Could you check a few things on this model? Use its own coordinates, in mm. A direction names the side the tool comes from. Round coordinates to 2 decimals unless told otherwise and drop trailing zeros. Loops run counter-clockwise (first coordinate to the right, second up) from the corner with the lowest first, then second, coordinate; pieces in that order, holes last. Notation, with made-up numbers: (46.25, 52.25) -> (67.25, 52.25) arc R12 cw to (67.25, 65.25) -> close; hole circle Ø7 at (9, -35.75). An arc over 180 degrees is marked (long way). One line per item, written item: value.
Autodesk Fusion 360 part; units mm, degrees
sketch "Skizze1" plane through (0, 0, 0) normal (0, 0, 1) x (1, 0, 0)
  line L0 (-90, -60) -> (90, -60)
  line L1 (90, -60) -> (90, 60)
  line L2 (90, 60) -> (-90, 60)
  line L3 (-90, 60) -> (-90, -60)
  line L4 (0, -120.4862) -> (0, 94.8054) construction
  line L5 (-128.125, 0) -> (128.8109, 0) construction
  line L6 (-75, 45) -> (75, 45)
  line L7 (75, 45) -> (75, -45)
  line L8 (75, -45) -> (-75, -45)
  line L9 (-75, -45) -> (-75, 45)
  point P0 (0, 60)
  point P1 (-90, 0)
  point P2 (-75, 45)
  point P3 (75, 45)
  point P4 (75, -45)
  point P5 (-75, -45)
  dimension "d1" = 120
  dimension "d2" = 180
  dimension "d3" = 15
  dimension "d4" = 15
  dimension "d5" = 15
  dimension "d6" = 15
extrude "Extrusion1" add sketch "Skizze1" along normal blind 50 contours L0 L1 L2 L3 | L6 L7 L8 L9
sketch "Skizze2" plane through (0, 0, 50) normal (0, 0, 1) x (-1, 0, 0)
  line L0 (90, -60) -> (90, 60)
  line L1 (90, 60) -> (-90, 60)
  line L2 (-90, 60) -> (-90, -60)
  line L3 (-90, -60) -> (90, -60)
  point P0 (-75, 45)
  point P1 (-75, -45)
  point P2 (75, -45)
  point P3 (75, 45)
hole "Bohrung1" at (-75, 45, 50) at (-75, -45, 50) at (75, -45, 50) at (75, 45, 50) direction (0, 0, -1) diameter 6.6 depth 50 tip angle 180 counterbore diameter 14.55 counterbore depth 40
(1) For pin 1 Ø8.5 at (x, y) = (75, 45) entering from -Z; pin 2 Ø7.5 at (x, y) = (74.5, 44) entering from +Z, each with a flat end and sliding along its axis, tell me the tip position at first contact or that it passes through.
Results below:
pin 1: stops at z = 0
pin 2: stops at z = 10
(2) Imagine slicing it at C-C on x = -75. Write out the boundary of the cut face in (y, z) (3 decimals), then the cut area to 3 significant figures.
Results below:
outline: (-60, 0) -> (-48.3, 0) -> (-48.3, 10) -> (-52.275, 10) -> (-52.275, 50) -> (-60, 50) -> close; (-41.7, 0) -> (41.7, 0) -> (41.7, 10) -> (37.725, 10) -> (37.725, 50) -> (-37.725, 50) -> (-37.725, 10) -> (-41.7, 10) -> close; (48.3, 0) -> (60, 0) -> (60, 50) -> (52.275, 50) -> (52.275, 10) -> (48.3, 10) -> close
area: 4,700 mm²
(3) We'd pull the mould along Y, two halves only. Please class faces 3 (the face through (-1, -60, 25)), 4 (the face through (1, 60, 25)), 5 (the face through (-73, 42, 10)), 6 (the face through (-1, 1, 50)): +Y half, -Y half, draft (parallel to the pull), parting line (faces both ways), or undercut.
Results below:
face 3: -Y half
face 4: +Y half
face 5: undercut
face 6: draft
(4) Imagine slicing it at B-B on z = 37.5. Write out the boundary of the cut face in (x, y) (3 decimals), then the cut area to 3 significant figures.
Results below:
outline: (-90, -60) -> (90, -60) -> (90, 60) -> (-90, 60) -> close; hole circle Ø14.55 at (-75, -45); hole circle Ø14.55 at (-75, 45); hole circle Ø14.55 at (75, -45); hole circle Ø14.55 at (75, 45)
area: 20,900 mm²
(5) Imagine slicing it at A-A on y = -45. Write out the boundary of the cut face in (x, z) (3 decimals), then the cut area to 3 significant figures.
Results below:
outline: (-90, 0) -> (-78.3, 0) -> (-78.3, 10) -> (-82.275, 10) -> (-82.275, 50) -> (-90, 50) -> close; (-71.7, 0) -> (71.7, 0) -> (71.7, 10) -> (67.725, 10) -> (67.725, 50) -> (-67.725, 50) -> (-67.725, 10) -> (-71.7, 10) -> close; (78.3, 0) -> (90, 0) -> (90, 50) -> (82.275, 50) -> (82.275, 10) -> (78.3, 10) -> close
area: 7,700 mm²
(6) On a 3-axis mill with a long thin cutter (end or side, diameter ignored), from which of +Z, -Z, +X, -X, +Y, -Y can I reach the whole of each face in a straight line? I mean faces 1 (the face through (77, -48, 10)), 2 (the face through (-77.23, 47.43, 4.93)). Say none if no direction works.
Results below:
face 1: +Z
face 2: +Z, -Z
(7) Please list where these lines run through material, in increasing order: L1, parallel to Y at x = 75, z = 4; L2, parallel to X at y = -45, z = 4.75; L3, parallel to Y at x = 75, z = 33 (3 decimals).
Results below:
L1: y = -60 to -48.3, -41.7 to 41.7, 48.3 to 60
L2: x = -90 to -78.3, -71.7 to 71.7, 78.3 to 90
L3: y = -60 to -52.275, -37.725 to 37.725, 52.275 to 60
